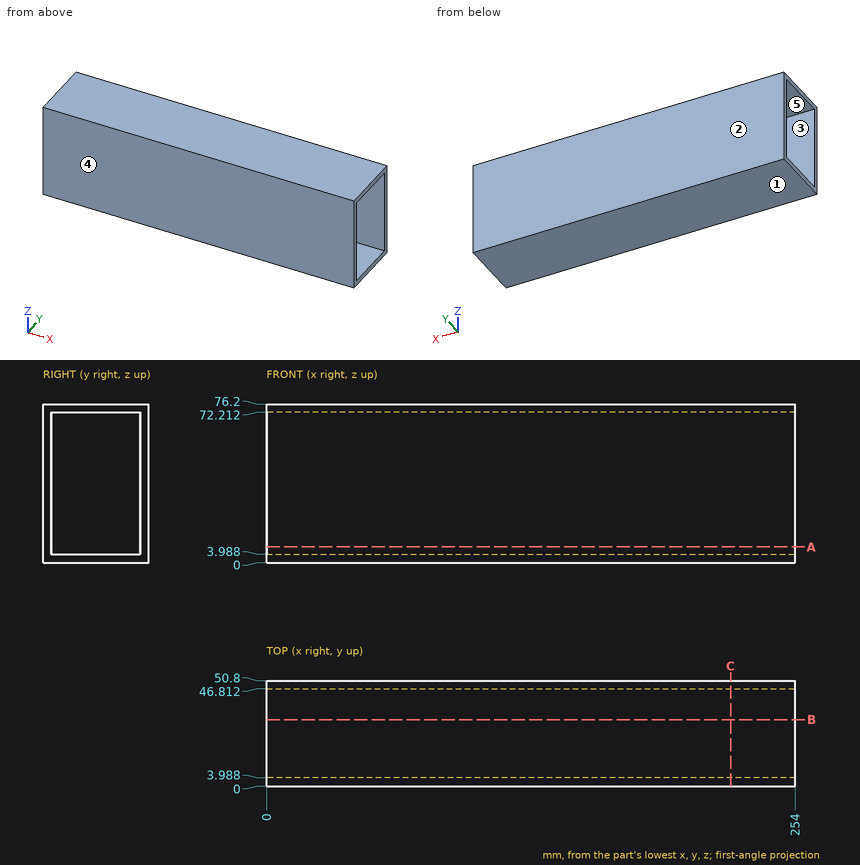
Geometry: see drawing. Coordinates: mm, zero at the bounding-box minimum. A direction names the side the tool comes from. Give positions to 0.01 mm unless a question says otherwise; leave off trailing zeros. Loops run counter-clockwise (first coordinate to the right, second up) from the corner with the lowest first, then second, coordinate; pieces in that order, holes last. Notation, with made-up numbers: (26.25, -30.5) - (57.25, -30.5) arc R16 ccw to (57.25, -8.5) - close; hole circle Ø1 at (70, 77.25). An arc over 180 degrees is marked (long way). Answer as CSV lines item,"result". Start each with the question number.
1. Pin query (flat end, axial travel): P1, Ø10, axis at y = 37, z = 22.5, coming from the -X side. Return the tip coordinate at first contact, or that it passes through.
2. Section B-B, the plane y = 32. Return loops of the section in (x, z), plus the area to 3 significant figures.
3. Reachability of the marked faces 4 and 5 from +Z, -Z, +X, -X, +Y, -Y: full face, straight path, thin tool, end or side. Return the list, or none.
4. Section A-A, the plane z = 7.5. Return loops of the section in (x, y).
5. Draft query along Y for the marked faces 1, 2 and 3. Return one class per face: released by +Y, released by -Y, zero draft, split by the parting line, or undercut.
6. Ray query, L1, parallel to Z at x = 56, y = 37.5; L2, parallel to Y at x = 195, z = 57.5. Return the intervals inside material, ascending.
7. Section C-C, the plane x = 223. Return loops of the section in (y, z).
Answers:
1,P1,"passes through"
2,outline,"(0, 0) - (254, 0) - (254, 3.99) - (0, 3.99) - close; (0, 72.21) - (254, 72.21) - (254, 76.2) - (0, 76.2) - close"
2,area,"2,030 mm2"
3,face 4,"+Z, -Z, +X, -X, -Y"
3,face 5,"+X, -X"
4,outline,"(0, 0) - (254, 0) - (254, 3.99) - (0, 3.99) - close; (0, 46.81) - (254, 46.81) - (254, 50.8) - (0, 50.8) - close"
5,face 1,"zero draft"
5,face 2,"released by +Y"
5,face 3,"undercut"
6,L1,"z = 0 to 3.99, 72.21 to 76.2"
6,L2,"y = 0 to 3.99, 46.81 to 50.8"
7,outline,"(0, 0) - (50.8, 0) - (50.8, 76.2) - (0, 76.2) - close; hole (3.99, 3.99) - (46.81, 3.99) - (46.81, 72.21) - (3.99, 72.21) - close"
